Work out the finished part from the listing and answer in its coordinate system (mm). A direction names the side the tool comes from. Round coordinates to 2 decimals unless told otherwise and drop trailing zeros. Write each loop counter-clockwise with the first axis right and the second up, starting at its lowest first coordinate (ties: lowest second). Pieces come first, ordered by that corner, then holes. Notation, with made-up numbers: (27, -35) - (36, -35) arc R31 cw to (36, 4) - close; hole circle Ø1 at (-23.75, 87). An arc over 180 degrees is marked (long way). Answer as a JSON object with one key per item and string values.
```python
from build123d import *

# Parameters (mm, degrees)
SKETCH1_W           = 28
SKETCH1_H           = 14.2
BOSS_EXTRUDE1_DEPTH = 33
SKETCH2_R           = 2.321908149
BOSS_EXTRUDE3_DEPTH = 4
SKETCH3_W           = 6.974752534
SKETCH3_H           = 3.176308394
BOSS_EXTRUDE4_DEPTH = 5
SKETCH4_W           = 5.77752576
SKETCH4_H           = 2.149777027
CUT_EXTRUDE1_DEPTH  = 5


with BuildPart() as part:
    # Sketch1 → Boss-Extrude1 (new body)
    with BuildSketch(Plane(origin=(0, 0, 0), x_dir=(1, 0, 0), z_dir=(0, 1, 0))):
        with Locations((-14, 7.1)):
            Rectangle(SKETCH1_W, SKETCH1_H)
    extrude(amount=BOSS_EXTRUDE1_DEPTH)

    # Sketch2 → Boss-Extrude3 (add)
    with BuildSketch(Plane(origin=(0, 33, 0), x_dir=(1, 0, 0), z_dir=(0, 1, 0))):
        with Locations(Location((-5.331542912, 7.506333926, 0), (0, 0, 270))):
            Circle(SKETCH2_R)
    extrude(amount=BOSS_EXTRUDE3_DEPTH)

    # Sketch3 → Boss-Extrude4 (add)
    with BuildSketch(Plane(origin=(0, 0, 0), x_dir=(0, 0, -1), z_dir=(1, 0, 0))):
        with Locations((7.1, 2.624490745)):
            Rectangle(SKETCH3_W, SKETCH3_H)
    extrude(amount=BOSS_EXTRUDE4_DEPTH)

    # Sketch4 → Cut-Extrude1 (cut)
    with BuildSketch(Plane(origin=(5, 0, 0), x_dir=(0, 0, -1), z_dir=(1, 0, 0))):
        with Locations((7.1, 2.467865933)):
            Rectangle(SKETCH4_W, SKETCH4_H)
    extrude(amount=-CUT_EXTRUDE1_DEPTH, mode=Mode.SUBTRACT)


solid = part.part
```
Item 1: Consider line 1 along X through (y, z) = (19.5, -5.5); line 2 along Y through (x, z) = (-11, -12.75); line 3 along Y through (x, z) = (2, -10.25). Determine where each line is inside the solid, lowest interval first.
Results found:
{"line 1": "-28 to 0", "line 2": "0 to 33", "line 3": "1.04 to 4.21"}
Item 2: Each of these flat-tipped pins is pushed along its axis until it touches: P1, Ø1.7, axis at x = 3.5, y = 2.5, coming from the -Z side; P2, Ø2.5, axis at x = 1.5, y = 2, coming from the +Z side; P3, Ø1, axis at x = -8.5, z = -7, coming from the +Y side. Where does it stop, or does it pass through?
Results found:
{"P1": "z = -10.59", "P2": "z = -3.61", "P3": "y = 33"}
Item 3: Determine the mould class of faces 1 (the flat face through (2, 1.036, -7)), 2 (the flat face through (2, 3, -3.613)), 3 (the flat face through (3, 2, -9.989)) for opening direction Z: pulls with the +Z half, pulls with the -Z half, needs draft (parallel to the pull), parting line crosses it, or undercut.
Results found:
{"face 1": "needs draft", "face 2": "pulls with the +Z half", "face 3": "undercut"}
Item 4: A cutting plane is placed at A-A (x = 2). Write down the section's boundary in (y, z), and give its area (3 significant figures).
Results found:
{"outline": "(1.04, -10.59) - (4.21, -10.59) - (4.21, -3.61) - (1.04, -3.61) - close; hole (1.39, -9.99) - (3.54, -9.99) - (3.54, -4.21) - (1.39, -4.21) - close", "area": "9.73 mm²"}
Item 5: A cutting plane is placed at B-B (x = -6.5). Write down the section's boundary in (y, z).
Results found:
{"outline": "(0, -14.2) - (33, -14.2) - (33, -9.51) - (37, -9.51) - (37, -5.5) - (33, -5.5) - (33, 0) - (0, 0) - close"}
Item 6: A cutting plane is placed at C-C (z = -12.25). Write down the section's boundary in (x, y).
Results found:
{"outline": "(-28, 0) - (0, 0) - (0, 33) - (-28, 33) - close"}
Item 7: A cutting plane is placed at D-D (y = 31). Write down the section's boundary in (x, z), and give its area (3 significant figures).
Results found:
{"outline": "(-28, -14.2) - (0, -14.2) - (0, 0) - (-28, 0) - close", "area": "398 mm²"}
Item 8: For faces 4 (the flat face through (2, 3, -10.587)), 5 (the cylindrical face through (-3.374, 34.972, -6.258)), 6 (the flat face through (2, 4.213, -7)), 7 (the flat face through (3, 2, -4.211)), determine the directions among +Z, -Z, +X, -X, +Y, -Y from which every point of the face is accessible in a straight line to the end or side of a thin tool.
Results found:
{"face 4": "-Z, +X, +Y, -Y", "face 5": "+Y", "face 6": "+Z, -Z, +X, +Y", "face 7": "+X"}
